from build123d import *

# Parameters (mm, degrees)
SKETCH1_W           = 15.5
SKETCH1_H           = 15.5
BOSS_EXTRUDE1_DEPTH = 15


with BuildPart() as part:
    # Sketch1 → Boss-Extrude1 (new body)
    with BuildSketch(Plane(origin=(0, 0, 0), x_dir=(1, 0, 0), z_dir=(0, 1, 0))):
        Rectangle(SKETCH1_W, SKETCH1_H)
    extrude(amount=BOSS_EXTRUDE1_DEPTH)

    # Sketch4 → Revolve5 (revolve)
    with BuildSketch(Plane.XY):
        with BuildLine():
            Line((9.2, 15), (0, 15))
            Line((0, 15), (0, 60))
            add(Edge.make_bspline(
                [(9.2, 15), (9.152248995, 24.690987366), (8.00981737, 34.882517262), (4.24723587, 50.506815958), (2.016778071, 56.805895624), (0, 60)],
                knots=[0, 0, 0, 0, 0.565414982, 0.665414982, 1, 1, 1, 1], degree=3))
        make_face()
    revolve(axis=Axis((0, 15, 0), (0, 1, 0)))


solid = part.part
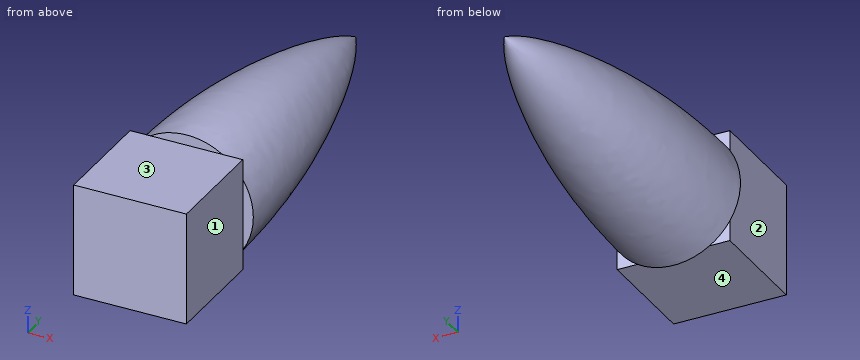
Design review of the part built by this model. Coordinates are the model's own, in mm. Face numbers are marked on the shaded views. A direction names the side the tool comes from. Give positions to 0.01 mm unless a question says otherwise; leave off trailing zeros. Order: outer loops, then holes, each group sorted by start corner. A loop starts at its lowest first (then second) coordinate and runs counter-clockwise, first axis right, second up. Notation, with made-up numbers: (-24.5, 25.25) - (-20.5, 25.25) arc R11 ccw to (-20.5, 34.25) - close; hole circle Ø8 at (35.5, 83). An arc over 180 degrees is marked (long way). Use CSV: the item, a comma, the result in double quotes. Start each with the question number.
Q1. Take a section at A-A (y = 4.5). State the section outline as (x, z) points, and give its area (3 significant figures).
Q2. Machinability: for the marked faces 1, 2, 3 and 4, which of the approach directions +Z, -Z, +X, -X, +Y, -Y give a long, thin tool a straight path to every point of the face, cutting with its end or side? Answer none if there is none.
Q3. For P1, Ø4.5, axis at x = 3, y = 11, coming from the -Z side; P2, Ø4.5, axis at y = 4, z = 0.5, coming from the -X side; P3, Ø1, axis at x = 3.5, y = 52, coming from the -Z side, all flat-tipped, find the tip position at first contact; note any pin that passes through.
Q4. For line 1 (Z direction, x = 2, y = 6.5); line 2 (Z direction, x = -0.5, y = 37), list the stretches that pass through material, from the lowest coordinate up.
Calculated:
1,outline,"(-7.75, -7.75) - (7.75, -7.75) - (7.75, 7.75) - (-7.75, 7.75) - close"
1,area,"240 mm²"
2,face 1,"+Z, -Z, +X, -Y"
2,face 2,"+Z, -Z, -X, -Y"
2,face 3,"+Z, +X, -X, -Y"
2,face 4,"-Z, +X, -X, -Y"
3,P1,"stops at z = -7.75"
3,P2,"stops at x = -7.75"
3,P3,"stops at z = -1.97"
4,line 1,"z = -7.75 to 7.75"
4,line 2,"z = -7.24 to 7.24"
